from build123d import *

# Parameters (mm, degrees)
SKETCH2_W           = 0.78
SKETCH2_H           = 1.5
SKETCH2_H_2         = 0.75
BOSS_EXTRUDE1_DEPTH = 1.56
SKETCH3_R           = 0.5
BOSS_EXTRUDE2_DEPTH = 14
SKETCH4_R           = 0.5
CUT_EXTRUDE1_DEPTH  = 14
SKETCH5_R           = 0.5
CUT_EXTRUDE2_DEPTH  = 14


with BuildPart() as part:
    # Sketch2 → Boss-Extrude1 (new body)
    with BuildSketch(Plane.XY):
        with Locations((0.39, -14.03)):
            Rectangle(SKETCH2_W, SKETCH2_H)
        with Locations((1.17, -14.03)):
            Rectangle(SKETCH2_W, SKETCH2_H)
        Polygon((0, 1.5), (0, 0.75), (0.78, 0.75), (0.78, 0), (1.56, 0), (1.56, 1.5), align=None)
        with Locations((0.39, 0.375)):
            Rectangle(SKETCH2_W, SKETCH2_H_2)
    extrude(amount=BOSS_EXTRUDE1_DEPTH)

    # Sketch3 → Boss-Extrude2 (add)
    with BuildSketch(Plane.XZ):
        with Locations(Location((0.78, 0.78, 0), (0, 0, 90))):
            Circle(SKETCH3_R)
    extrude(amount=BOSS_EXTRUDE2_DEPTH)

    # Sketch4 → Cut-Extrude1 (cut)
    with BuildSketch(Plane.ZY):
        with Locations((0.799406884, 0.75)):
            Circle(SKETCH4_R)
    extrude(amount=-CUT_EXTRUDE1_DEPTH, mode=Mode.SUBTRACT)

    # Sketch5 → Cut-Extrude2 (cut)
    with BuildSketch(Plane.ZY):
        with Locations((0.78, -14.03)):
            Circle(SKETCH5_R)
    extrude(amount=-CUT_EXTRUDE2_DEPTH, mode=Mode.SUBTRACT)


solid = part.part
Source: CAD feature listing. Evaluate the final solid. Frame: model axes, mm. A direction names the side the tool comes from. Coordinates: 2 decimals unless noted, no trailing zeros. Loops run counter-clockwise (first coordinate to the right, second up) from the corner with the lowest first, then second, coordinate; pieces in that order, holes last. Notation, with made-up numbers: (37, 37.25) - (78, 37.25) arc R24 cw to (78, 52.25) - close; hole circle Ø11 at (17, -11.5). An arc over 180 degrees is marked (long way). Return JSON: item names as keys, results as strings.
Q1. Section B-B, the plane z = 0.7. Return loops of the section in (x, y).
Results:
{"outline": "(0, -14.78) - (1.56, -14.78) - (1.56, -14.52) - (0, -14.52) - close; (0, -13.54) - (1.56, -13.54) - (1.56, -13.28) - (1.27, -13.28) - (1.27, 0) - (1.56, 0) - (1.56, 0.26) - (0, 0.26) - (0, 0) - (0.29, 0) - (0.29, -13.28) - (0, -13.28) - close; (0, 1.24) - (1.56, 1.24) - (1.56, 1.5) - (0, 1.5) - close"}
Q2. Access query for faces 5 (the cylindrical face through (0.63, -6.547, 1.257)), 6 (the flat face through (1, 1.5, 1)). Directions: +Z, -Z, +X, -X, +Y, -Y. A direction counts if a zero-diameter tool reaches every point of the face in a straight line with its end or side. Return the directions, or none.
Results:
{"face 5": "none", "face 6": "+Z, -Z, +X, -X, +Y"}
Q3. Section C-C, the plane x = 0.78. Return loops of the section in (y, z).
Results:
{"outline": "(-14.78, 0) - (-13.28, 0) - (-13.28, 0.28) - (0, 0.28) - (0, 0) - (1.5, 0) - (1.5, 1.56) - (0, 1.56) - (0, 1.28) - (-13.28, 1.28) - (-13.28, 1.56) - (-14.78, 1.56) - close; hole circle Ø1 at (-14.03, 0.78); hole circle Ø1 at (0.75, 0.8)"}
Q4. Section D-D, the plane y = -5.5. Return loops of the section in (x, z).
Results:
{"outline": "circle Ø1 at (0.78, 0.78)"}
Q5. Material intervals for line 1 along Y through (x, z) = (1.05, 0.78); line 2 along Y through (x, z) = (0.8, 0.55); line 3 along Y through (x, z) = (0.65, 1.4), sorted ascending.
Results:
{"line 1": "-14.78 to -14.53, -13.53 to 0.25, 1.25 to 1.5", "line 2": "-14.78 to -14.47, -13.59 to 0.32, 1.18 to 1.5", "line 3": "-14.78 to -13.28, 0 to 1.5"}
Q6. Section A-A, the plane y = -14.03. Return loops of the section in (x, z).
Results:
{"outline": "(0, 0) - (1.56, 0) - (1.56, 0.28) - (0, 0.28) - close; (0, 1.28) - (1.56, 1.28) - (1.56, 1.56) - (0, 1.56) - close"}
Q7. Mould query, pull axis Z, two halves, no side actions, for faces 1 (the cylindrical face through (0.769, -13.534, 0.715)), 2 (the cylindrical face through (0.769, 0.262, 0.691)), 3 (the flat face through (1, -14, 1.56)), 4 (the flat face through (1, -14.78, 1)). Classes: released by +Z, released by -Z, zero draft, split by the parting line, or undercut.
Results:
{"face 1": "undercut", "face 2": "undercut", "face 3": "released by +Z", "face 4": "zero draft"}
